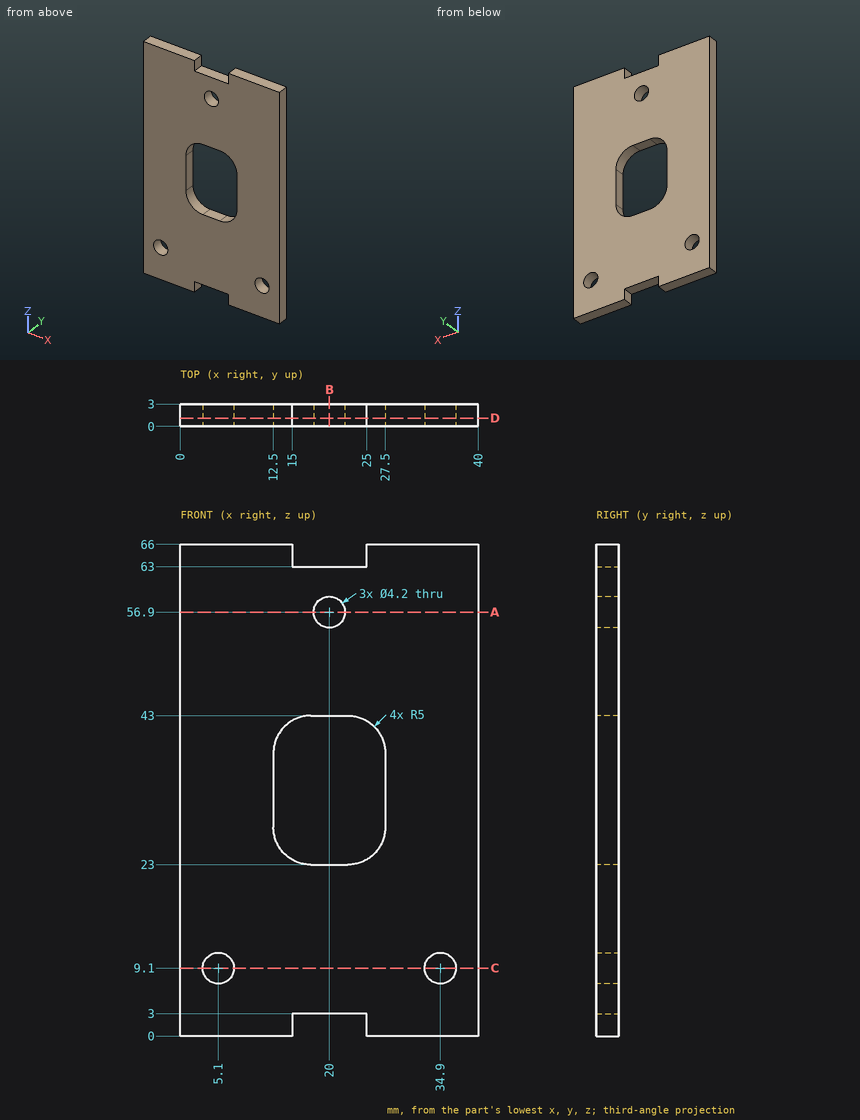
Drawing for the job (mm, zero at the part's lowest x, y, z). Coordinates: 2 decimals unless noted, no trailing zeros. Write each loop counter-clockwise with the first axis right and the second up, starting at its lowest first coordinate (ties: lowest second). Pieces come first, ordered by that corner, then holes. Notation, with made-up numbers: (41.5, 78.5) - (85.5, 78.5) arc R22 cw to (85.5, 95.5) - close; hole circle Ø10 at (49.5, -18). An arc over 180 degrees is marked (long way). Write each question's results on one line, items separated by ' | '. Start each with the question number.
1) Cut at D-D (y = 1.1). Write the cut outline in (x, z).
2) Cut at C-C (z = 9.1). Write the cut outline in (x, y), then the cut area to 3 significant figures.
3) Cut at A-A (z = 56.9). Write the cut outline in (x, y).
4) Probe line 1 along X through (y, z) = (1.6, 9.1); line 2 along X through (y, z) = (2.05, 56.9); line 3 along Z through (x, y) = (22.5, 0.4). List the from-to ranges inside material, lowest first. Write a range as from..to.
5) Flat gauge pins, fed straight in: P1, Ø0.9, axis at x = 19.5, y = 1, coming from the +Z side; P2, Ø0.9, axis at x = 21.5, y = 1.5, coming from the -Z side; P3, Ø3.5, axis at x = 34.9, z = 9.1, coming from the +Y side. Where does each tip first touch, or does it go through?
6) Cut at B-B (x = 20). Write the cut outline in (y, z), then the cut area to 3 significant figures.
Returned:
1) outline: (0, 0) - (15, 0) - (15, 3) - (25, 3) - (25, 0) - (40, 0) - (40, 66) - (25, 66) - (25, 63) - (15, 63) - (15, 66) - (0, 66) - close; hole circle Ø4.2 at (5.1, 9.1); hole (12.5, 28) arc R5 ccw to (17.5, 23) - (22.5, 23) arc R5 ccw to (27.5, 28) - (27.5, 38) arc R5 ccw to (22.5, 43) - (17.5, 43) arc R5 ccw to (12.5, 38) - close; hole circle Ø4.2 at (20, 56.9); hole circle Ø4.2 at (34.9, 9.1)
2) outline: (0, 0) - (3, 0) - (3, 3) - (0, 3) - close; (7.2, 0) - (32.8, 0) - (32.8, 3) - (7.2, 3) - close; (37, 0) - (40, 0) - (40, 3) - (37, 3) - close | area: 94.8 mm^2
3) outline: (0, 0) - (17.9, 0) - (17.9, 3) - (0, 3) - close; (22.1, 0) - (40, 0) - (40, 3) - (22.1, 3) - close
4) line 1: 0..3, 7.2..32.8, 37..40 | line 2: 0..17.9, 22.1..40 | line 3: 3..23, 43..63
5) P1: z = 63 | P2: z = 3 | P3: through
6) outline: (0, 3) - (3, 3) - (3, 23) - (0, 23) - close; (0, 43) - (3, 43) - (3, 54.8) - (0, 54.8) - close; (0, 59) - (3, 59) - (3, 63) - (0, 63) - close | area: 107 mm^2
